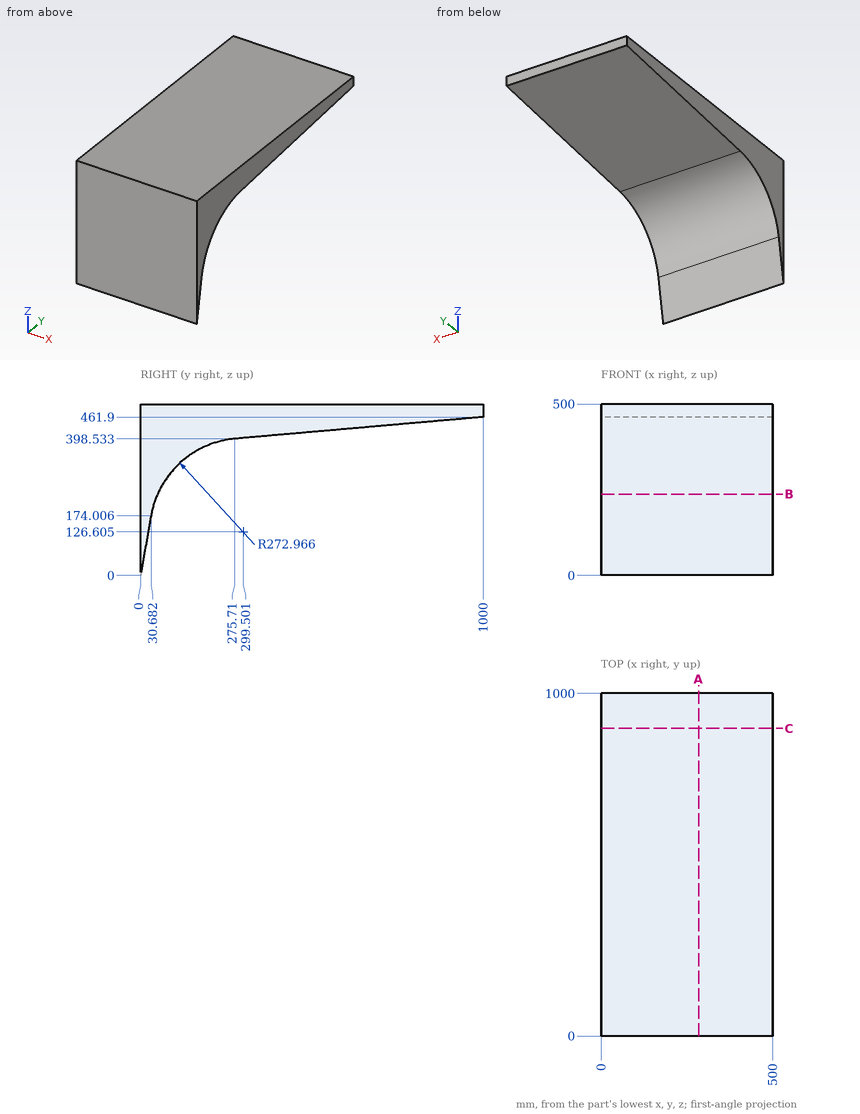
Geometry: see drawing. Coordinates: mm, zero at the bounding-box minimum. Coordinates: 2 decimals unless noted, no trailing zeros. Write each loop counter-clockwise with the first axis right and the second up, starting at its lowest first coordinate (ties: lowest second). Pieces come first, ordered by that corner, then holes. Notation, with made-up numbers: M 41.25,23.25 L 84.25,23.25 A9 ccw 84.25,36.25 Z; hole C 46,-23 d11. An arc over 180 degrees is marked long. Answer as a JSON object with one key per item and string values.
1. Cut plane A-A on x = 284.5. Output: boundary loops of the cut face in (y, z) (1 decimal), plus the area to 3 significant figures.
Evaluation:
{"outline": "M 0,0 L 30.7,174 A273 cw 275.7,398.5 L 1000,461.9 L 1000,500 L 0,500 Z", "area": "103,000 mm^2"}
2. Contact query for flat-ended pins moving along their axis: P1, Ø4, axis at x = 403.5, y = 245, coming from the -Z side; P2, Ø6, axis at x = 289.5, y = 233.5, coming from the -Z side. Output: stop coordinate, or through.
Evaluation:
{"P1": "z = 393.66", "P2": "z = 390.71"}
3. Cut plane C-C on y = 897.5. Output: boundary loops of the cut face in (x, z).
Evaluation:
{"outline": "M 0,452.93 L 500,452.93 L 500,500 L 0,500 Z"}
4. Cut plane B-B on z = 237. Output: boundary loops of the cut face in (x, y) (1 decimal), plus the area to 3 significant figures.
Evaluation:
{"outline": "M 0,0 L 500,0 L 500,49.9 L 0,49.9 Z", "area": "24,900 mm^2"}
5. Ray query, L1, parallel to Y at x = 369, z = 165.5; L2, parallel to Z at x = 452.5, y = 443.5; L3, parallel to Z at x = 74, y = 859 (1 decimal). Return the intervals inside material, ascending.
Evaluation:
{"L1": "0 to 29.18", "L2": "413.21 to 500", "L3": "449.6 to 500"}
